Geometry check sheet. Reference: the model listing, model coordinates, mm. Give positions to 0.01 mm unless a question says otherwise; leave off trailing zeros. Write each loop counter-clockwise with the first axis right and the second up, starting at its lowest first coordinate (ties: lowest second). Pieces come first, ordered by that corner, then holes. Notation, with made-up numbers: M 36,53 L 55,53 A15 ccw 55,72 Z; hole C 13.5,53.5 d10. An arc over 180 degrees is marked long. Use one line per item in the form item = value. Start each with the question number.
```python
from build123d import *

# Parameters (mm, degrees)
F0_R     = 2.5
F0_R_2   = 52.5
F1_DEPTH = 30
F3_DEPTH = 120.001
F4_R     = 3


with BuildPart() as f1:
    # F0 (on Top) → F1 (new body)
    with BuildSketch(Plane.XY):
        with BuildLine():
            ThreePointArc((0, 10), (2.928932, 2.928932), (10, 0))
            Line((10, 0), (110, 0))
            ThreePointArc((110, 0), (117.071068, 2.928932), (120, 10))
            Line((120, 10), (120, 110))
            ThreePointArc((120, 110), (117.071068, 117.071068), (110, 120))
            Line((110, 120), (10, 120))
            ThreePointArc((10, 120), (2.928932, 117.071068), (0, 110))
            Line((0, 110), (0, 10))
        make_face()
        with Locations((7.6, 7.6)):
            Circle(F0_R, mode=Mode.SUBTRACT)
        with Locations((112.4, 7.6)):
            Circle(F0_R, mode=Mode.SUBTRACT)
        with Locations((60, 60)):
            Circle(F0_R_2, mode=Mode.SUBTRACT)
        with Locations((7.6, 112.4)):
            Circle(F0_R, mode=Mode.SUBTRACT)
        with Locations((112.4, 112.4)):
            Circle(F0_R, mode=Mode.SUBTRACT)
    extrude(amount=F1_DEPTH)

    # F2 (on face) → F3 (cut, through all)
    with BuildSketch(Plane.YZ.offset(120)):
        Polygon((0, 45), (0, 2), (114, 21), (117.5, 0), (125, 0), (125, 45), (120, 45), align=None)
    extrude(amount=-F3_DEPTH, mode=Mode.SUBTRACT)

    # F4
    f4_edges = [f1.edges().sort_by_distance(p)[0] for p in [
        (7.5, 60, 0),
    ]]
    fillet(f4_edges, radius=F4_R)


solid = f1.part
```
(1) Depth check by flat-ended pin: pin 1 (6 mm diameter, centred on x = 24.5, z = 7.5, fed in from +Y); pin 2 (10 mm diameter, centred on x = 21, y = 42.5, fed in from -Z); pin 3 (10 mm diameter, centred on x = 16.5, z = 6.5, fed in from +Y); pin 4 (5 mm diameter, centred on x = 37.5, z = 15, fed in from -Y). Enter the tip coordinate at first touch or a pass-through.
(2) Sectioned sample at B-B, the plane y = 60. Record the boundary of the cut face in (x, z).
(3) Thickness scan on probe 1 along X at (y, z) = (60, 9.25); probe 2 along X at (y, z) = (43.5, 6.75); probe 3 along Z at (x, y) = (99.5, 98). Record the ranges inside material, lowest first. Write a range as [from, to].
(4) Sectioned sample at A-A, the plane x = 60. Record the boundary of the cut face in (y, z), plus the area to 3 significant figures.
(5) Draft check along Y on faces 1 (the flat face through (120, 70, 8)), 2 (the cylindrical face through (118, 4, 1)), 3 (the cylindrical face through (111.86, 109.96, 10.35)). Enter one of: released by +Y, released by -Y, zero draft, split by the parting line, or undercut.
Numbers:
q1.pin_1 = 116.75
q1.pin_2 = through
q1.pin_3 = 117.25
q1.pin_4 = 106.17
q2.outline = M 0,0 L 4.5,0 A3 ccw 7.5,3 L 7.5,12 L 0,12 Z; M 112.5,3 A3 ccw 115.5,0 L 120,0 L 120,12 L 112.5,12 Z
q3.probe_1 = [0, 7.5], [112.5, 120]
q3.probe_2 = [0, 10.16], [109.84, 120]
q3.probe_3 = [0.08, 18.33]
q4.outline = M 0,0 L 4.5,0 A3 ccw 7.5,3 L 7.5,3.25 L 0,2 Z; M 112.5,3 A3 ccw 115.5,0 L 117.5,0 L 114,21 L 112.5,20.75 Z
q4.area = 83.9 mm2
q5.face_1 = zero draft
q5.face_2 = released by -Y
q5.face_3 = undercut
